CAD build for the part. Positions are in the model's coordinates, mm. Coordinates: 2 decimals unless noted, no trailing zeros. Write item = value, one per line. Start each with the question number.
(1) Flat gauge pin, fed straight in: P1, Ø3, axis at x = 2.35, y = 30.69, coming from the -Z side. Where does the tip first touch, or does it go through?
(2) Pull direction Y, two halves, no side cores. Call faces 1 (the face through (2, -4.309, -1)), 2 (the face through (1.813, -1.814, -0.935)), 3 (the face through (38.352, 30, -1)): +Y half, -Y half, draft (parallel to the pull), parting line (faces both ways), or undercut.
(3) Drill centre lines: line 1 (Y direction, x = 1, z = -1.6); line 2 (X direction, y = 61, z = -1.8); line 3 (X direction, y = 62, z = -1.4). Where is each one in solid material? Low to high. Write a range as from..to.
```python
from build123d import *

# Parameters (mm, degrees)
SKETCH1_W          = 72
SKETCH1_H          = 70
BASE_FLANGE1_DEPTH = 1.89738
SKETCH6_R          = 2.5
SKETCH6_R_2        = 2
CUT_EXTRUDE1_DEPTH = 2


# Sheet-metal steps are written as plain solids
with BuildPart() as part:
    # Sketch1 → Base-Flange1 (new body)
    with BuildSketch(Plane.XY):
        with Locations((2.352272727, 30.691243667)):
            Rectangle(SKETCH1_W, SKETCH1_H)
    extrude(amount=-BASE_FLANGE1_DEPTH)

    # Sketch6 → Cut-Extrude1 (cut)
    with BuildSketch(Plane.XY):
        with Locations((2.354647746, 60.626948244)):
            Circle(SKETCH6_R)
        with Locations((2.354647746, 0.626948244)):
            Circle(SKETCH6_R)
        with Locations((2.354647746, 30.691243667)):
            Circle(SKETCH6_R_2)
    extrude(amount=-CUT_EXTRUDE1_DEPTH, mode=Mode.SUBTRACT)


solid = part.part
```
Findings below:
q1.P1 = through
q2.face_1 = -Y half
q2.face_2 = undercut
q2.face_3 = draft
q3.line_1 = -4.31..-1.47, 2.73..29.22, 32.16..58.53, 62.73..65.69
q3.line_2 = -33.65..-0.12, 4.83..38.35
q3.line_3 = -33.65..0.27, 4.44..38.35
